Read the model definition and answer for the solid it produces. Units are mm, in the model's axes. A direction names the side the tool comes from. Round coordinates to 2 decimals unless told otherwise and drop trailing zeros. Order: outer loops, then holes, each group sorted by start corner. A loop starts at its lowest first (then second) coordinate and runs counter-clockwise, first axis right, second up.
from build123d import *

# Parameters (mm, degrees)
F1_DEPTH = 3.175
F3_DEPTH = 9.525
F4_R     = 1.8034
F5_DEPTH = 149.861


with BuildPart() as f1:
    # F0 (on Right) → F1 (new body)
    with BuildSketch(Plane.YZ):
        Polygon((-48.322902, 60.276262), (-48.322902, -41.323738), (101.537098, 9.476262), (101.537098, 60.276262), align=None)
    extrude(amount=F1_DEPTH)

    # F2 (on face) → F3 (join)
    with BuildSketch(Plane.YZ.offset(3.175)):
        Polygon((-48.322902, 57.101262), (-48.322902, -41.323738), (-45.147902, -41.323738), (-45.147902, 57.101262), (98.362098, 57.101262), (98.362098, 9.476262), (101.537098, 9.476262), (101.537098, 57.101262), (101.537098, 60.276262), (-48.322902, 60.276262), align=None)
    extrude(amount=F3_DEPTH)

    # F4 (on face) → F5 (cut, through all)
    with BuildSketch(Plane.XZ.offset(48.322902)):
        with Locations((6.35, -34.973738)):
            Circle(F4_R)
        with Locations((6.35, -22.273738)):
            Circle(F4_R)
        with Locations((6.35, -9.573738)):
            Circle(F4_R)
        with Locations((6.35, 3.126262)):
            Circle(F4_R)
        with Locations((6.35, 15.826262)):
            Circle(F4_R)
        with Locations((6.35, 28.526262)):
            Circle(F4_R)
        with Locations((6.35, 41.226262)):
            Circle(F4_R)
        with Locations((6.35, 53.926262)):
            Circle(F4_R)
    extrude(amount=-F5_DEPTH, mode=Mode.SUBTRACT)


solid = f1.part
Q1. For faces 4 (the face through (8, -45.148, 7)), 5 (the face through (8, 100, 9.476)), 6 (the face through (6.115, 99.927, 55.714)), determine the directions among +Z, -Z, +X, -X, +Y, -Y from which every point of the face is accessible in a straight line to the end or side of a thin tool.
Outcome:
face 4: -Z, +X
face 5: -Z, +X, +Y
face 6: +Y, -Y
Q2. Flat-ended cylindrical pins translate along their axes: pin 1 (3 mm diameter, centred on x = 6.35, z = 28.53, fed in from -Y); pin 2 (2 mm diameter, centred on x = 9.5, z = -22.5, fed in from +Y); pin 3 (3 mm diameter, centred on x = 9, y = 7.5, fed in from -Z); pin 4 (5 mm diameter, centred on y = -23.5, z = -9.5, fed in from +X) (3 decimals). Find the tip coordinate at first contact, or state that the pin passes through.
Outcome:
pin 1: passes through
pin 2: stops at y = -45.15
pin 3: stops at z = 57.1
pin 4: stops at x = 3.175
Q3. Straight lines are drawn through the part: probe 1 along Z at (x, y) = (6.35, 100.95); probe 2 along Y at (x, z) = (11.5, 30); probe 3 along Y at (x, z) = (10.5, -12). For each, find the intervals that lie inside material, in ascending order.
Outcome:
probe 1: z = 9.48 to 14.02, 17.63 to 26.72, 30.33 to 39.42, 43.03 to 52.12, 55.73 to 60.28
probe 2: y = -48.32 to -45.15, 98.36 to 101.54
probe 3: y = -48.32 to -45.15
Q4. A cutting plane is placed at A-A, the plane z = 11.5. Give the vertices of the cut face in (x, y) (3 decimals).
Outcome:
outline: (0, -48.323) - (12.7, -48.323) - (12.7, -45.148) - (3.175, -45.148) - (3.175, 98.362) - (12.7, 98.362) - (12.7, 101.537) - (0, 101.537) - close
Q5. A cutting plane is placed at C-C, the plane y = -17.5. Give the vertices of the cut face in (x, z) (3 decimals).
Outcome:
outline: (0, -30.875) - (3.175, -30.875) - (3.175, 57.101) - (12.7, 57.101) - (12.7, 60.276) - (0, 60.276) - close
Q6. A cutting plane is placed at D-D, the plane y = 34.5. Give the vertices of the cut face in (x, z) (3 decimals), plus the area to 3 significant figures.
Outcome:
outline: (0, -13.248) - (3.175, -13.248) - (3.175, 57.101) - (12.7, 57.101) - (12.7, 60.276) - (0, 60.276) - close
area: 264 mm2
Q7. A cutting plane is placed at B-B, the plane x = 10. Give the vertices of the cut face in (y, z).
Outcome:
outline: (-48.32, -41.32) - (-45.15, -41.32) - (-45.15, 57.1) - (98.36, 57.1) - (98.36, 9.48) - (101.54, 9.48) - (101.54, 60.28) - (-48.32, 60.28) - close
Q8. For a pull along X with two mould halves and no side action, classify faces 1 (the face through (0, 26, 21)), 2 (the face through (6.115, -46.758, 4.914)), 3 (the face through (1.57, 25.56, -16.28)) as released by +X, released by -X, zero draft, split by the parting line, or undercut.
Outcome:
face 1: released by -X
face 2: undercut
face 3: zero draft
